Drawing for the job (mm, zero at the part's lowest x, y, z). A direction names the side the tool comes from. Give positions to 0.01 mm unless a question says otherwise; leave off trailing zeros. Order: outer loops, then holes, each group sorted by start corner. A loop starts at its lowest first (then second) coordinate and runs counter-clockwise, first axis right, second up. Notation, with made-up numbers: (-22.75, 55.5) - (3.25, 55.5) arc R37 ccw to (3.25, 94.5) - close; hole circle Ø3 at (-34, -24.75). An arc over 180 degrees is marked (long way). One line per item, written item: value.
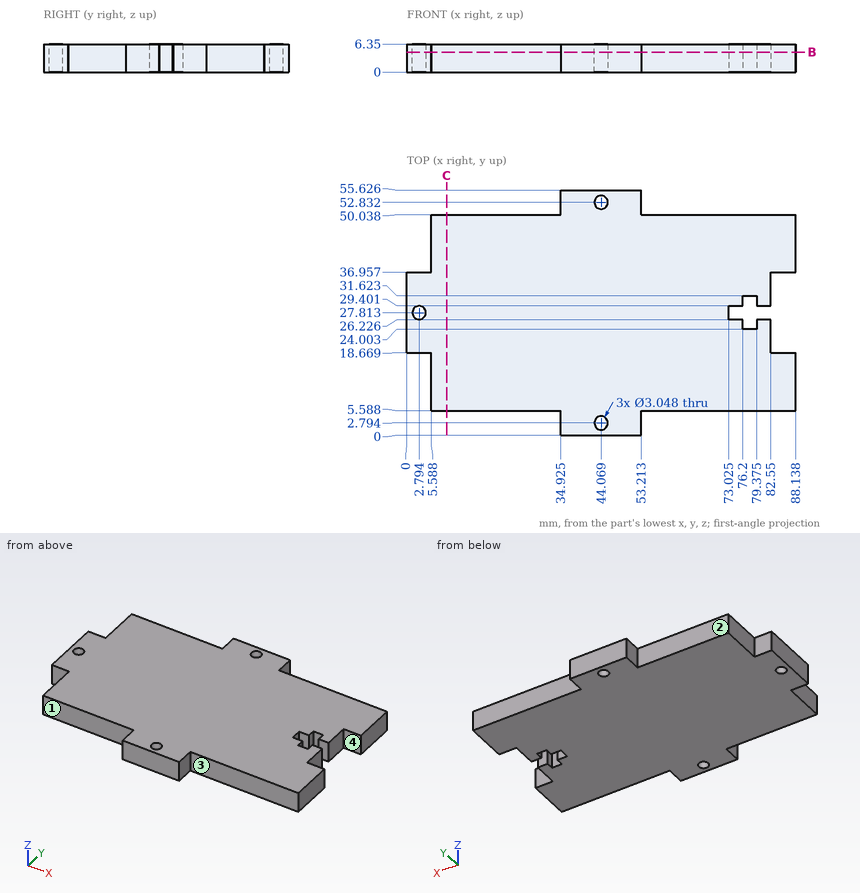
(1) Slice it at B-B, the plane z = 4.5. Count the separate pieces of the cut face and the enclosed holes in it, and give its area (3 significant figures).
Completed:
separate pieces: 1
enclosed holes: 3
area: 3,810 mm²
(2) 3-axis set-ups, long thin cutter, end or side, ignore diameter. For the marked faces 1, 2, 3 and 4: which of +Z, -Z, +X, -X, +Y, -Y reach the whole face in a straight line?
Completed:
face 1: +Z, -Z, -X, -Y
face 2: +Z, -Z, -X, +Y
face 3: +Z, -Z, +X, -Y
face 4: +Z, -Z, +X
(3) Pin check, flat tips, straight feed: P1, Ø2.5, axis at y = 25.5, z = 4.5, coming from the +X side; P2, Ø3, axis at y = 41.5, z = 3, coming from the -X side; P3, Ø1.9, axis at x = 14, z = 2, coming from the -Y side. Stop position of each tip, or through.
Completed:
P1: x = 82.55
P2: x = 5.59
P3: y = 5.59
(4) Drill centre lines: line 1 (Y direction, x = 85, z = 6); line 2 (Y direction, x = 43, z = 2) (1 decimal); line 3 (Y direction, x = 79.5, z = 1.5) (1 decimal). Where is each one in solid material? Low to high.
Completed:
line 1: 5.59 to 18.67, 36.96 to 50.04
line 2: 0 to 1.7, 3.9 to 51.7, 53.9 to 55.6
line 3: 5.6 to 26.2, 29.4 to 50
(5) Slice it at C-C, the plane x = 9. Give the cut face in (y, z).
Completed:
outline: (5.59, 0) - (50.04, 0) - (50.04, 6.35) - (5.59, 6.35) - close
